The listing builds one solid part. Answer for the finished solid, in the listing's coordinates (mm). A direction names the side the tool comes from. Round coordinates to 2 decimals unless told otherwise and drop trailing zeros. Write each loop counter-clockwise with the first axis right and the second up, starting at its lowest first coordinate (ties: lowest second). Pieces come first, ordered by that corner, then holes.
(1) Each of these flat-tipped pins is pushed along its axis until it touches: pin 1 Ø3.5 at (y, z) = (78, 3) entering from -X; pin 2 Ø3.5 at (y, z) = (78.5, 2) entering from +X; pin 3 Ø1 at (x, z) = (-3.5, 6) entering from -Y. Where does it stop, or does it pass through?
(2) A cutting plane is placed at A-A, the plane x = -0.25. Give the vertices of the cut face in (y, z), and give its area (3 significant figures).
(3) For faces 1 (the face through (6.84, 75, 2)), 2 (the face through (1, 75, 4.244)), 3 (the face through (2.19, -14.79, -2.3)), determine the directions among +Z, -Z, +X, -X, +Y, -Y from which every point of the face is accessible in a straight line to the end or side of a thin tool.
(4) A cutting plane is placed at D-D, the plane x = 8.5. Give the vertices of the cut face in (y, z), and give its area (3 significant figures).
(5) A cutting plane is placed at C-C, the plane y = 71.5. Give the vertices of the cut face in (x, z).
(6) Find the intervals of material crossed by probe 1 along Y at (x, z) = (10.5, 4.75); probe 2 along Y at (x, z) = (-2.75, -0.5); probe 3 along Z at (x, y) = (-2.25, -9.5), in increasing order.
(7) A cutting plane is placed at B-B, the plane z = 1.75. Give the vertices of the cut face in (x, y).
from build123d import *

# Parameters (mm, degrees)
SKETCH_1_W      = 26.5
SKETCH_1_H      = 11.5
EXTRUDE_1_DEPTH = 68.5
SKETCH_2_W      = 12
SKETCH_2_H      = 4.5
EXTRUDE_2_DEPTH = 14
SKETCH_3_R      = 4.5
EXTRUDE_3_DEPTH = 30


with BuildPart() as part:
    # 草图1 → 凸台-拉伸1 (new body)
    with BuildSketch(Plane(origin=(0, 0, 0), x_dir=(1, 0, 0), z_dir=(0, 1, 0))):
        with Locations((0.83974359, -1.993589744)):
            Rectangle(SKETCH_1_W, SKETCH_1_H)
    extrude(amount=EXTRUDE_1_DEPTH)

    # 草图2 → 凸台-拉伸2 (add)
    with BuildSketch(Plane(origin=(0, 68.5, 0), x_dir=(1, 0, 0), z_dir=(0, 1, 0))):
        with Locations((0.83974359, -1.993589744)):
            Rectangle(SKETCH_2_W, SKETCH_2_H)
    extrude(amount=EXTRUDE_2_DEPTH)

    # 草图3 → 凸台-拉伸3 (add)
    with BuildSketch(Plane.XZ):
        with Locations(Location((0.83974359, 1.993589744, 0), (0, 0, 270))):
            Circle(SKETCH_3_R)
    extrude(amount=EXTRUDE_3_DEPTH)


solid = part.part
Solutions:
1. pin 1: stops at x = -5.16
1. pin 2: stops at x = 6.84
1. pin 3: stops at y = 0
2. outline: (-30, -2.37) - (0, -2.37) - (0, -3.76) - (68.5, -3.76) - (68.5, -0.26) - (82.5, -0.26) - (82.5, 4.24) - (68.5, 4.24) - (68.5, 7.74) - (0, 7.74) - (0, 6.36) - (-30, 6.36) - close
2. area: 1,110 mm2
3. face 1: +Z, -Z, +X, +Y
3. face 2: +Z, +X, -X, +Y
3. face 3: -Y
4. outline: (0, -3.76) - (68.5, -3.76) - (68.5, 7.74) - (0, 7.74) - close
4. area: 788 mm2
5. outline: (-5.16, -0.26) - (6.84, -0.26) - (6.84, 4.24) - (-5.16, 4.24) - close
6. probe 1: y = 0 to 68.5
6. probe 2: y = -30 to 68.5
6. probe 3: z = -1.28 to 5.27
7. outline: (-12.41, 0) - (-3.65, 0) - (-3.65, -30) - (5.33, -30) - (5.33, 0) - (14.09, 0) - (14.09, 68.5) - (6.84, 68.5) - (6.84, 82.5) - (-5.16, 82.5) - (-5.16, 68.5) - (-12.41, 68.5) - close
